The model under review builds one solid part; all positions refer to its coordinate system, in mm. Round coordinates to 2 decimals unless told otherwise and drop trailing zeros. Write each loop counter-clockwise with the first axis right and the second up, starting at its lowest first coordinate (ties: lowest second). Pieces come first, ordered by that corner, then holes. Notation, with made-up numbers: (12, 36.25) - (71, 36.25) arc R26 ccw to (71, 61.25) - close; hole circle Ø6 at (88, 89.25). An arc over 180 degrees is marked (long way). Write each question's results on one line, items separated by ' | '.
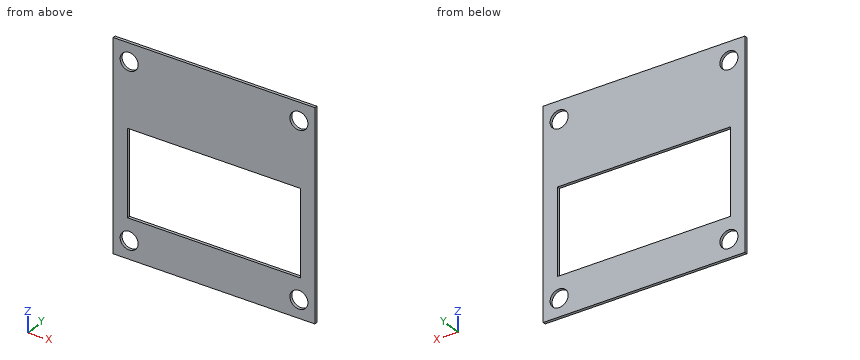
```python
from build123d import *

# Parameters (mm, degrees)
ESQUISSE1_W             = 28
ESQUISSE1_H             = 29
ESQUISSE1_W_2           = 24
ESQUISSE1_H_2           = 12
BOSS_EXTRU_1_DEPTH      = 0.4
ESQUISSE2_R             = 1.25
ENL_V_MAT_EXTRU_1_DEPTH = 10


with BuildPart() as part:
    # Esquisse1 → Boss.-Extru.1 (new body)
    with BuildSketch(Plane(origin=(0, 0, 0), x_dir=(1, 0, 0), z_dir=(0, 1, 0))):
        Rectangle(ESQUISSE1_W, ESQUISSE1_H)
        with Locations((0, 3)):
            Rectangle(ESQUISSE1_W_2, ESQUISSE1_H_2, mode=Mode.SUBTRACT)
    extrude(amount=BOSS_EXTRU_1_DEPTH)

    # Esquisse2 → Enlèv. mat.-Extru.1 (cut)
    with BuildSketch(Plane.XZ):
        with Locations(Location((11.78, -11.99, 0), (0, 0, 270))):
            Circle(ESQUISSE2_R)
        with Locations(Location((-11.78, 11.99, 0), (0, 0, 270))):
            Circle(ESQUISSE2_R)
        with Locations(Location((11.78, 11.99, 0), (0, 0, 270))):
            Circle(ESQUISSE2_R)
        with Locations(Location((-11.78, -11.99, 0), (0, 0, 270))):
            Circle(ESQUISSE2_R)
    extrude(amount=-ENL_V_MAT_EXTRU_1_DEPTH, mode=Mode.SUBTRACT)


solid = part.part
```
Q1. For probe 1 along X at (y, z) = (0.35, 11.99); probe 2 along Z at (x, y) = (6.25, 0.35); probe 3 along X at (y, z) = (0.2, -5), list the stretches that pass through material, from the lowest coordinate up.
Evaluation:
probe 1: x = -14 to -13.03, -10.53 to 10.53, 13.03 to 14 | probe 2: z = -14.5 to -9, 3 to 14.5 | probe 3: x = -14 to -12, 12 to 14
Q2. We need section B-B (x = 9). State the section outline as (y, z) points, plus the area to 3 significant figures.
Evaluation:
outline: (0, -14.5) - (0.4, -14.5) - (0.4, -9) - (0, -9) - close; (0, 3) - (0.4, 3) - (0.4, 14.5) - (0, 14.5) - close | area: 6.80 mm^2
Q3. We need section A-A (z = -11.99). State the section outline as (x, y) points, plus the area to 3 significant figures.
Evaluation:
outline: (-14, 0) - (-13.03, 0) - (-13.03, 0.4) - (-14, 0.4) - close; (-10.53, 0) - (10.53, 0) - (10.53, 0.4) - (-10.53, 0.4) - close; (13.03, 0) - (14, 0) - (14, 0.4) - (13.03, 0.4) - close | area: 9.20 mm^2
Q4. We need section C-C (y = 0.1). State the section outline as (x, z) points.
Evaluation:
outline: (-14, -14.5) - (14, -14.5) - (14, 14.5) - (-14, 14.5) - close; hole circle Ø2.5 at (-11.78, -11.99); hole circle Ø2.5 at (-11.78, 11.99); hole (-12, -9) - (12, -9) - (12, 3) - (-12, 3) - close; hole circle Ø2.5 at (11.78, -11.99); hole circle Ø2.5 at (11.78, 11.99)
